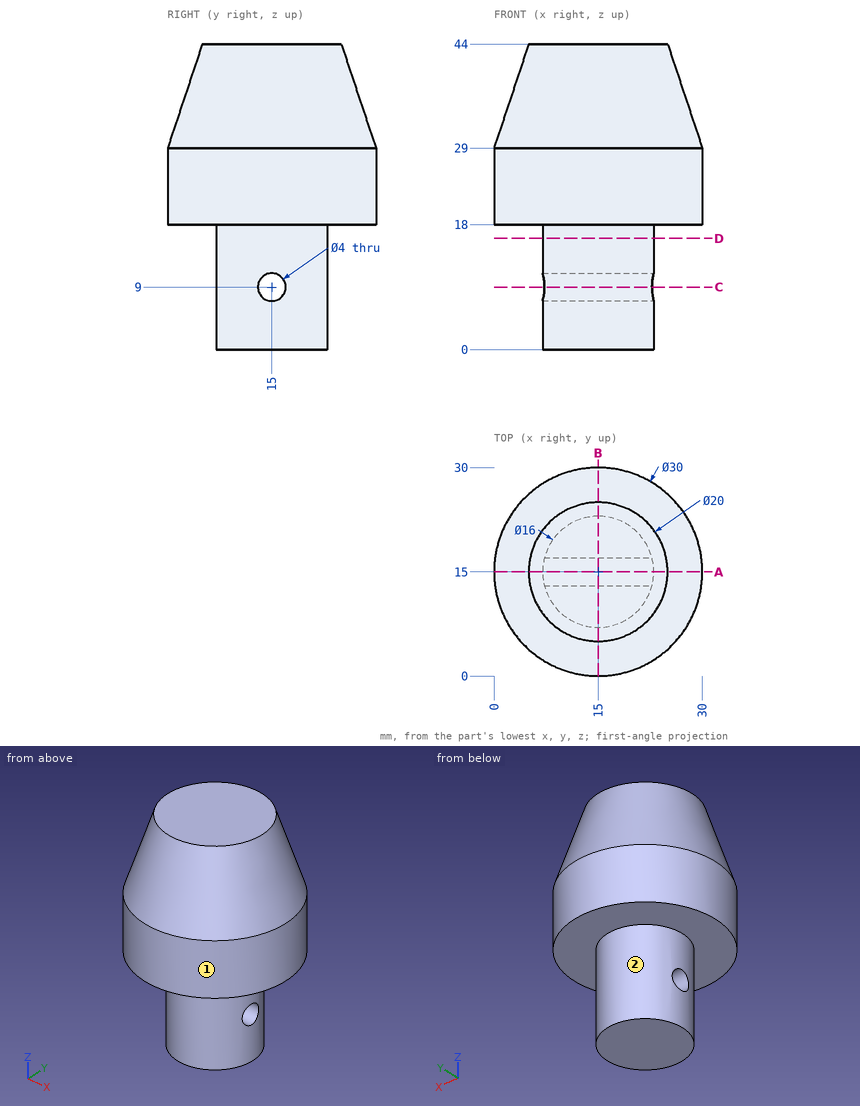
Answer from the drawing. Dimensions are ordinates in mm from the lowest x, y and z of the part. A direction names the side the tool comes from. Give positions to 0.01 mm unless a question says otherwise; leave off trailing zeros. Order: outer loops, then holes, each group sorted by start corner. A loop starts at its lowest first (then second) coordinate and runs counter-clockwise, first axis right, second up. Notation, with made-up numbers: (40.25, 19) -> (76.25, 19) arc R17 cw to (76.25, 52) -> close; hole circle Ø4 at (17, 68.25). An arc over 180 degrees is marked (long way). One line per item, written item: value. Start each with the question number.
(1) The part is cut by section A-A (y = 15). Determine the outline of the cut face in (x, z), and give its area (3 significant figures).
(2) The part is cut by section D-D (z = 16). Determine the outline of the cut face in (x, y).
(3) The part is cut by section C-C (z = 9). Determine the outline of the cut face in (x, y), and give its area (3 significant figures).
(4) The part is cut by section B-B (x = 15). Determine the outline of the cut face in (y, z).
(5) Straight lines are drawn through the part: L1, parallel to Z at x = 18.25, y = 15; L2, parallel to Y at x = 15, z = 9; L3, parallel to Y at x = 19.5, z = 9. For each, find the intervals that lie inside material, in ascending order.
(6) Flat-ended cylindrical pins translate along their axes: P1, Ø5, axis at x = 15, y = 5.5, coming from the -Z side; P2, Ø4, axis at y = 26, z = 29.5, coming from the -X side; P3, Ø6.5, axis at y = 15, z = 9, coming from the -X side; P4, Ø6, axis at x = 8.5, z = 27.5, coming from the +Y side. Find the tip coordinate at first contact, or state that the pin passes through.
(7) A tool of negligible diameter and unlimited length cuts with its end or side. For the marked faces 1 and 2, from which of +Z, -Z, +X, -X, +Y, -Y can it reach the whole face along a straight path? Write none if from no direction.
Taken from the geometry:
1. outline: (0, 18) -> (7, 18) -> (7, 11) -> (23, 11) -> (23, 18) -> (30, 18) -> (30, 29) -> (25, 44) -> (5, 44) -> (0, 29) -> close; (7, 0) -> (23, 0) -> (23, 7) -> (7, 7) -> close
1. area: 929 mm^2
2. outline: circle Ø16 at (15, 15)
3. outline: (7.25, 13) arc R8 ccw to (22.75, 13) -> close; (7.25, 17) -> (22.75, 17) arc R8 ccw to start
3. area: 138 mm^2
4. outline: (0, 18) -> (7, 18) -> (7, 0) -> (23, 0) -> (23, 18) -> (30, 18) -> (30, 29) -> (25, 44) -> (5, 44) -> (0, 29) -> close; hole circle Ø4 at (15, 9)
5. L1: 0 to 7, 11 to 44
5. L2: 7 to 13, 17 to 23
5. L3: 8.39 to 13, 17 to 21.61
6. P1: z = 0
6. P2: x = 3.05
6. P3: x = 7
6. P4: y = 29.59
7. face 1: +Z, -Z
7. face 2: -Z
